Check sheet for the modelled part. Datum: model origin and axes. Units: mm. Give positions to 0.01 mm unless a question says otherwise; leave off trailing zeros. Order: outer loops, then holes, each group sorted by start corner. A loop starts at its lowest first (then second) coordinate and runs counter-clockwise, first axis right, second up. Notation, with made-up numbers: (82, 0.5) - (118, 0.5) arc R23 ccw to (118, 26.5) - close; hole circle Ø6 at (21, -34.5). An arc over 180 degrees is marked (long way). Answer in a Markdown table with one row per item.
from build123d import *

# Parameters (mm, degrees)
F1_DEPTH = 5
F2_R     = 1.5
F3_DEPTH = 5


with BuildPart() as f1:
    # F0 (on Front) → F1 (new body)
    with BuildSketch(Plane.XZ):
        Polygon((90, -75), (125, -75), (125, 75), (-125, 75), (-125, -75), (-90, -75), (-90, -175), (90, -175), align=None)
    extrude(amount=F1_DEPTH)

    # F2 (on face) → F3 (cut)
    with BuildSketch(Plane.XZ.offset(5)):
        with Locations((0, 65)):
            Circle(F2_R)
        with Locations((-10, 45)):
            Circle(F2_R)
        with Locations((10, 45)):
            Circle(F2_R)
        with Locations((-84, -169)):
            Circle(F2_R)
        with Locations((-84, -144)):
            Circle(F2_R)
        with Locations((-84, -119)):
            Circle(F2_R)
        with Locations((-69, -169)):
            Circle(F2_R)
        with Locations((-69, -144)):
            Circle(F2_R)
        with Locations((-69, -119)):
            Circle(F2_R)
        with Locations((84, -169)):
            Circle(F2_R)
        with Locations((84, -144)):
            Circle(F2_R)
        with Locations((69, -169)):
            Circle(F2_R)
        with Locations((69, -119)):
            Circle(F2_R)
        with Locations((69, -144)):
            Circle(F2_R)
        with Locations((84, -119)):
            Circle(F2_R)
    extrude(amount=-F3_DEPTH, mode=Mode.SUBTRACT)


solid = f1.part
(1) Cross-section at B-B, the plane x = 110. Record the cut outline in (y, z), then the cut area to 3 significant figures.
Geometry says:
| item | result |
|---|---|
| outline | (-5, -75) - (0, -75) - (0, 75) - (-5, 75) - close |
| area | 750 mm² |
(2) Gauge pin test, flat ends, axial feed: P1, Ø2.5, axis at x = -106, y = -3, coming from the -Z side; P2, Ø12, axis at x = 95, z = -113.5, coming from the +Y side; P3, Ø2.5, axis at x = -69, z = -144, coming from the +Y side; P4, Ø1.5, axis at y = -3, z = -139, coming from the +X side. Record the tip position at first contact, or that the pin passes through.
Geometry says:
| item | result |
|---|---|
| P1 | z = -75 |
| P2 | y = 0 |
| P3 | through |
| P4 | x = 90 |
(3) Cross-section at C-C, the plane z = -136. Record the cut outline in (x, y).
Geometry says:
| item | result |
|---|---|
| outline | (-90, -5) - (90, -5) - (90, 0) - (-90, 0) - close |
(4) Thickness scan on L1, parallel to Z at x = -69, y = -2.2; L2, parallel to X at y = -1.35, z = -119; L3, parallel to Z at x = 83.5, y = -1.35. Record the ranges inside material, lowest first.
Geometry says:
| item | result |
|---|---|
| L1 | -175 to -170.5, -167.5 to -145.5, -142.5 to -120.5, -117.5 to 75 |
| L2 | -90 to -85.5, -82.5 to -70.5, -67.5 to 67.5, 70.5 to 82.5, 85.5 to 90 |
| L3 | -175 to -170.41, -167.59 to -145.41, -142.59 to -120.41, -117.59 to 75 |
(5) Cross-section at A-A, the plane y = -0.9. Give the number of separate pieces and of enclosed holes in the cut face, then the cut area to 3 significant figures.
Geometry says:
| item | result |
|---|---|
| separate pieces | 1 |
| enclosed holes | 15 |
| area | 55,400 mm² |
